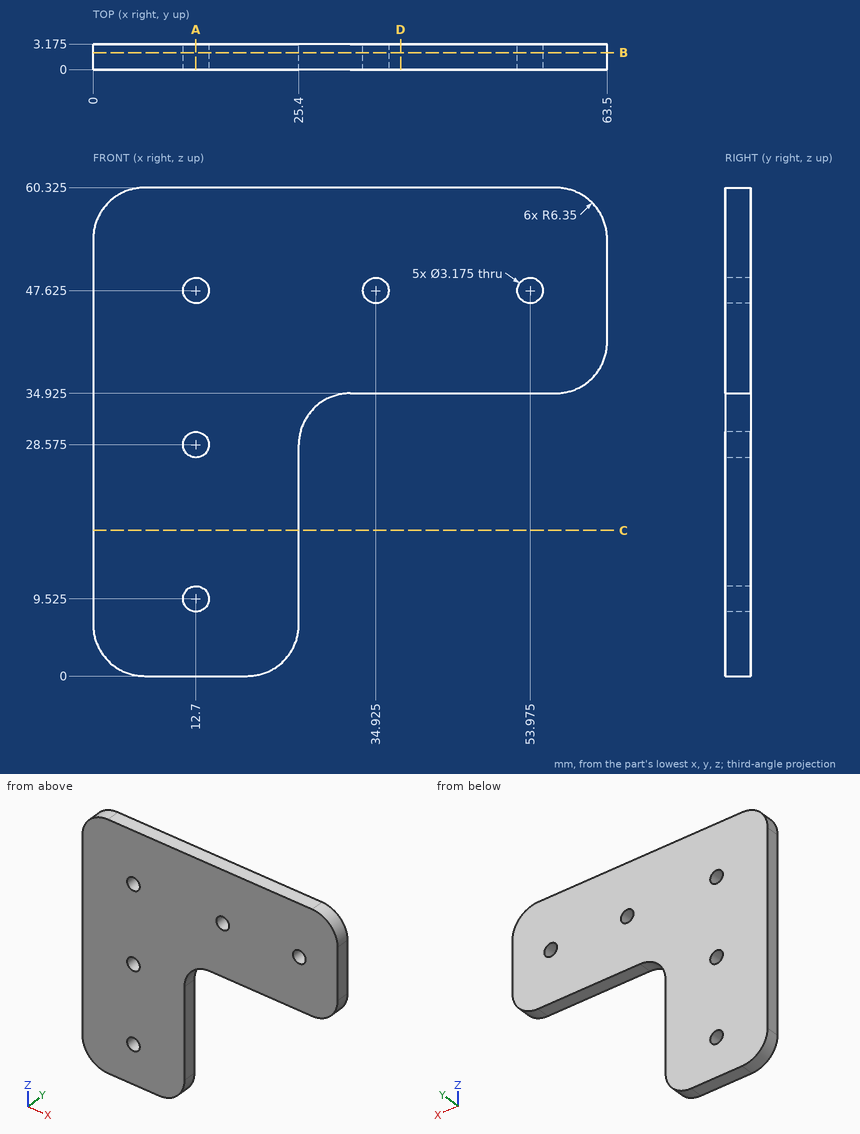
The figure shows three views and two pictorial views of one solid part (mm, origin at its lowest corner). Answer the questions. Round coordinates to 2 decimals unless told otherwise and drop trailing zeros. Loops run counter-clockwise (first coordinate to the right, second up) from the corner with the lowest first, then second, coordinate; pieces in that order, holes last. Notation, with made-up numbers: (-10.75, 80) - (-2.75, 80) arc R17 ccw to (-2.75, 105) - close; hole circle Ø1 at (13.25, 49). An arc over 180 degrees is marked (long way). Use one line per item in the form item = value. Start each with the question number.
(1) Find section A-A on x = 12.7. Determine the outline of the cut face in (y, z) (1 decimal).
(2) Find section C-C on z = 18. Determine the outline of the cut face in (x, y) (3 decimals), and give its area (3 significant figures).
(3) Find section B-B on y = 2.1. Give the number of separate pieces and of enclosed holes in the cut face, and give its area (3 significant figures).
(4) Find section D-D on x = 38. Determine the outline of the cut face in (y, z) (3 decimals).
(5) Consider line 1 (Z direction, x = 12.7, y = 2.2) (1 decimal); line 2 (Z direction, x = 38, y = 0.4) (3 decimals); line 3 (X direction, y = 2.1, z = 21.5). Determine where each line is inside the solid, lowest interval first.
Answer list:
q1.outline = (0, 0) - (3.2, 0) - (3.2, 7.9) - (0, 7.9) - close; (0, 11.1) - (3.2, 11.1) - (3.2, 27) - (0, 27) - close; (0, 30.2) - (3.2, 30.2) - (3.2, 46) - (0, 46) - close; (0, 49.2) - (3.2, 49.2) - (3.2, 60.3) - (0, 60.3) - close
q2.outline = (0, 0) - (25.4, 0) - (25.4, 3.175) - (0, 3.175) - close
q2.area = 80.6 mm^2
q3.separate_pieces = 1
q3.enclosed_holes = 5
q3.area = 2,430 mm^2
q4.outline = (0, 34.925) - (3.175, 34.925) - (3.175, 60.325) - (0, 60.325) - close
q5.line_1 = 0 to 7.9, 11.1 to 27, 30.2 to 46, 49.2 to 60.3
q5.line_2 = 34.925 to 60.325
q5.line_3 = 0 to 25.4
